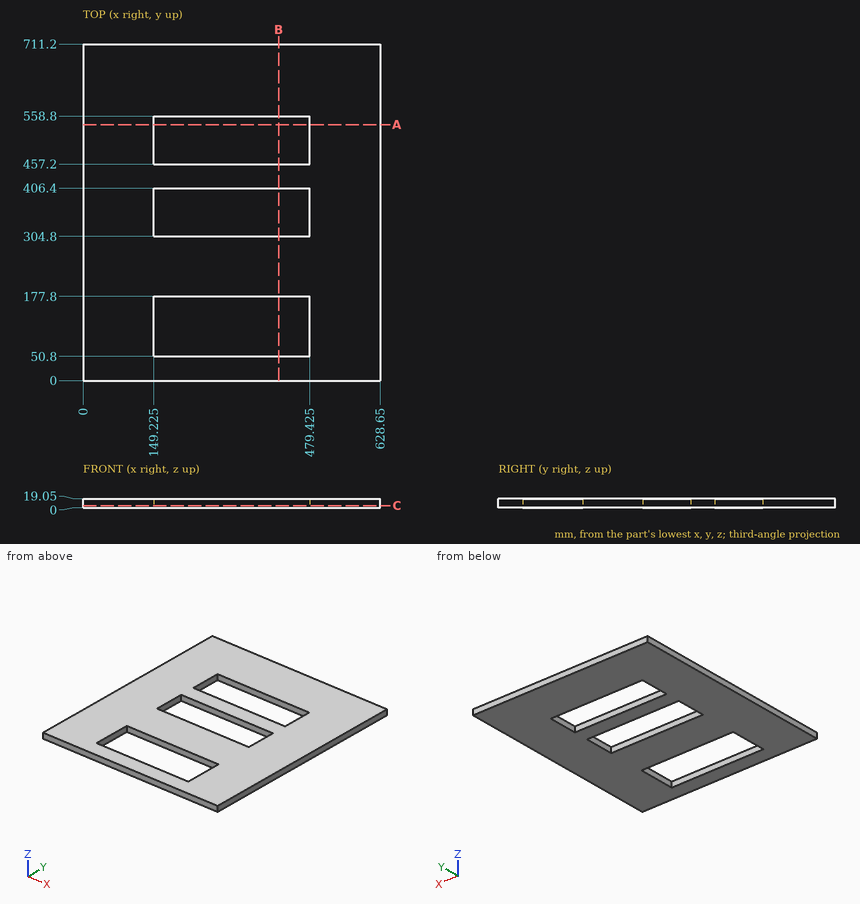
Geometry: see drawing. Coordinates: mm, zero at the bounding-box minimum. Round coordinates to 2 decimals unless told otherwise and drop trailing zeros. Loops run counter-clockwise (first coordinate to the right, second up) from the corner with the lowest first, then second, coordinate; pieces in that order, holes last. Notation, with made-up numbers: M 79,79.25 L 112,79.25 A23 cw 112,108.25 Z; hole C 39.25,37 d6. An arc over 180 degrees is marked long. Use a Markdown table: item, result. Add a question column.
1. Cut plane B-B, the plane x = 413.5. Output: boundary loops of the cut face in (y, z), and give its area (3 significant figures).
2. Contact query for a flat-ended pin moving along its axis: pin 1 (2 mm diameter, centred on y = 188, z = 11.5, fed in from -X). Output: stop coordinate, or through.
3. Cut plane A-A, the plane y = 541. Output: boundary loops of the cut face in (x, z) (3 decimals).
4. Cut plane C-C, the plane z = 4. Output: boundary loops of the cut face in (x, y) (3 decimals).
5. Ray query, line 1 along Y through (x, z) = (257, 4); line 2 along X through (y, z) = (391.5, 16.5) (3 decimals). Return the intervals inside material, ascending. Write a range as [from, to].
Solution:
| question | item | result |
|---|---|---|
| 1 | outline | M 0,0 L 50.8,0 L 50.8,19.05 L 0,19.05 Z; M 177.8,0 L 304.8,0 L 304.8,19.05 L 177.8,19.05 Z; M 406.4,0 L 457.2,0 L 457.2,19.05 L 406.4,19.05 Z; M 558.8,0 L 711.2,0 L 711.2,19.05 L 558.8,19.05 Z |
| 1 | area | 7,260 mm2 |
| 2 | pin 1 | stops at x = 0 |
| 3 | outline | M 0,0 L 149.225,0 L 149.225,19.05 L 0,19.05 Z; M 479.425,0 L 628.65,0 L 628.65,19.05 L 479.425,19.05 Z |
| 4 | outline | M 0,0 L 628.65,0 L 628.65,711.2 L 0,711.2 Z; hole M 149.225,50.8 L 479.425,50.8 L 479.425,177.8 L 149.225,177.8 Z; hole M 149.225,304.8 L 479.425,304.8 L 479.425,406.4 L 149.225,406.4 Z; hole M 149.225,457.2 L 479.425,457.2 L 479.425,558.8 L 149.225,558.8 Z |
| 5 | line 1 | y = [0, 50.8], [177.8, 304.8], [406.4, 457.2], [558.8, 711.2] |
| 5 | line 2 | x = [0, 149.225], [479.425, 628.65] |
